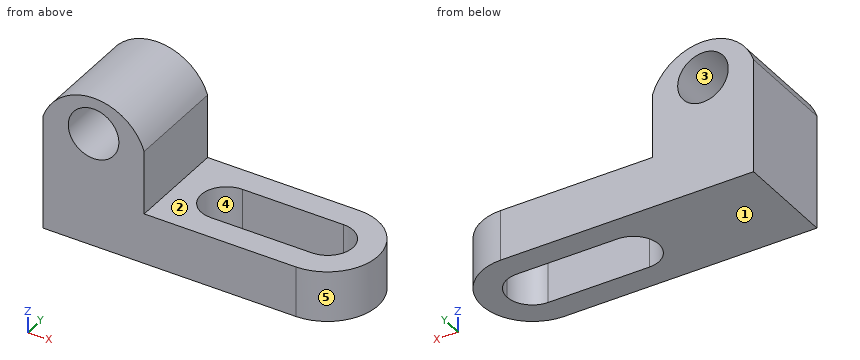
```python
from build123d import *

# Parameters (mm, degrees)
F0_R     = 6.35
F1_DEPTH = 25.4
F3_DEPTH = 25.4
F5_DEPTH = 25.4


with BuildPart() as f1:
    # F0 (on Front) → F1 (new body)
    with BuildSketch(Plane.XZ):
        with BuildLine():
            Line((0, 28.6947377026), (0, 0))
            Line((0, 0), (76.2, 0))
            Line((76.2, 0), (76.2, 12.7))
            Line((76.2, 12.7), (25.4, 12.7))
            Line((25.4, 12.7), (25.4, 28.6947377026))
            ThreePointArc((25.4, 28.6947377026), (12.7, 37.8535239462), (0, 28.6947377026))
        make_face()
        with Locations((12.7, 28.6947377026)):
            Circle(F0_R, mode=Mode.SUBTRACT)
    extrude(amount=F1_DEPTH)

    # F2 (on face) → F3 (cut)
    with BuildSketch(Plane.XY.offset(12.7)):
        with BuildLine():
            ThreePointArc((38.1, -6.3605568116), (42.5901280605, -8.220428751), (44.45, -12.7105568116))
            ThreePointArc((44.45, -12.7105568116), (42.5901280605, -17.2006848721), (38.1, -19.0605568116))
            Line((38.1, -19.0605568116), (38.1, -19.0711169188))
            Line((38.1, -19.0711169188), (63.5052786794, -19.0499978059))
            Line((63.5052786794, -19.0499978059), (63.5, -6.3499994515))
            Line((63.5, -6.3499994515), (38.1, -6.3605568116))
        make_face()
        with BuildLine():
            Line((38.1, -19.0605568116), (38.1, -6.3605568116))
            ThreePointArc((38.1, -6.3605568116), (31.75, -12.7105568116), (38.1, -19.0605568116))
        make_face()
        with BuildLine():
            ThreePointArc((38.1, -19.0605568116), (42.5901280605, -17.2006848721), (44.45, -12.7105568116))
            ThreePointArc((44.45, -12.7105568116), (42.5901280605, -8.220428751), (38.1, -6.3605568116))
            Line((38.1, -6.3605568116), (38.1, -19.0605568116))
        make_face()
        with BuildLine():
            ThreePointArc((69.85, -12.7), (67.9901280605, -8.2098719395), (63.5, -6.35))
            ThreePointArc((63.5, -6.35), (57.1500005485, -12.7026393399), (63.5052786794, -19.0499978059))
            ThreePointArc((63.5052786794, -19.0499978059), (67.9919939678, -17.1882613775), (69.85, -12.7))
        make_face()
    extrude(amount=-F3_DEPTH, mode=Mode.SUBTRACT)

    # F4 (on face) → F5 (cut)
    with BuildSketch(Plane.XY.offset(12.7)):
        with BuildLine():
            ThreePointArc((63.4973606602, 0), (76.1177273109, -12.7), (63.4973606602, -25.4))
            Line((63.4973606602, -25.4), (76.2, -25.4))
            Line((76.2, -25.4), (76.2, 0))
            Line((76.2, 0), (63.4973606602, 0))
        make_face()
    extrude(amount=-F5_DEPTH, mode=Mode.SUBTRACT)


solid = f1.part
```
The model under review builds one solid part; all positions refer to its coordinate system, in mm. Face numbers are marked on the shaded views. A direction names the side the tool comes from. Round coordinates to 2 decimals unless told otherwise and drop trailing zeros. Write each loop counter-clockwise with the first axis right and the second up, starting at its lowest first coordinate (ties: lowest second). Pieces come first, ordered by that corner, then holes.
(1) Machinability: for the marked faces 1 and 2, which of the approach directions +Z, -Z, +X, -X, +Y, -Y give a long, thin tool a straight path to every point of the face, cutting with its end or side? Answer none if there is none.
(2) Wall thickness on L1, parallel to Y at x = 43, z = 11.5; L2, parallel to Z at x = 26, y = -3.25; L3, parallel to X at y = -12.5, z = 8: over which ranges is each line inside the solid? List them lowest first.
(3) Mouldability with a two-part tool opening along Y and no side actions: class the marked faces 3, 4 and 5 as +Y half, -Y half, draft (parallel to the pull), parting line (faces both ways), or undercut.
(4) We need section D-D on z = 29.5. Give the boundary of the cut face in (x, y).
(5) Insertion check: pin 1 (12 mm diameter, centred on x = 44.5, y = -6, fed in from +Z); pin 2 (10 mm diameter, centred on y = -17.5, z = 21, fed in from +X). Each pin has a flat end and moves straight along its axis. Give the tip position at first contact, or say it passes through.
(6) We need section A-A on x = 12.7. Give the boundary of the cut face in (y, z).
(7) We need section B-B on y = -9. Give the boundary of the cut face in (x, z).
Findings below:
1. face 1: -Z, +X, -X, +Y, -Y
1. face 2: +Z, +X, +Y, -Y
2. L1: y = -25.4 to -19.07, -6.36 to 0
2. L2: z = 0 to 12.7
2. L3: x = 0 to 31.75, 69.85 to 76.12
3. face 3: draft
3. face 4: undercut
3. face 5: parting line
4. outline: (0.3, -25.4) - (6.4, -25.4) - (6.4, 0) - (0.3, 0) - close; (19, -25.4) - (25.1, -25.4) - (25.1, 0) - (19, 0) - close
5. pin 1: stops at z = 12.7
5. pin 2: stops at x = 25.4
6. outline: (-25.4, 0) - (0, 0) - (0, 22.34) - (-25.4, 22.34) - close; (-25.4, 35.04) - (0, 35.04) - (0, 37.85) - (-25.4, 37.85) - close
7. outline: (0, 0) - (32.95, 0) - (32.95, 12.7) - (25.4, 12.7) - (25.4, 28.69) arc R13.38 ccw to (0, 28.69) - close; (68.66, 0) - (75.57, 0) - (75.57, 12.7) - (68.66, 12.7) - close; hole circle Ø12.7 at (12.7, 28.69)
